Read the model definition and answer for the solid it produces. Units are mm, in the model's axes. A direction names the side the tool comes from. Give positions to 0.01 mm unless a question says otherwise; leave off trailing zeros. Order: outer loops, then holes, each group sorted by start corner. A loop starts at its lowest first (then second) coordinate and runs counter-clockwise, first axis right, second up. Notation, with made-up numbers: (35.25, 5.5) -> (89.25, 5.5) arc R25 cw to (89.25, 23.5) -> close; hole circle Ø10 at (5.5, 13). An arc over 180 degrees is marked (long way). Answer as CSV lines item,"result". Start each with the question number.
1) For faces 5 (the face through (-59.09, -59.46, 0.49)), 6 (the face through (-49, -57.4, 0.5)), determine the directions among +Z, -Z, +X, -X, +Y, -Y from which every point of the face is accessible in a straight line to the end or side of a thin tool.
2) Find section A-A (z = 0.15). State how many separate pieces and enclosed holes the cut face has, and give its area (3 significant figures).
3) The mould has two halves that part along Y. Classify faces 1 (the face through (59.328, -57.995, 0.493)), 2 (the face through (-49, -49.1, 0.5)), 3 (the face through (31, -48, 1)), 4 (the face through (-33, -49, 0.5)): +Y half, -Y half, draft (parallel to the pull), parting line (faces both ways), or undercut.
4) Find section C-C (y = -48). Determine the outline of the cut face in (x, z), and give its area (3 significant figures).
5) Find section D-D (x = 37). Determine the outline of the cut face in (y, z).
6) Flat-ended cylindrical pins translate along their axes: pin 1 Ø0.5 at (y, z) = (-46.5, 0.5) entering from +X; pin 2 Ø0.5 at (x, z) = (-15, 0.5) entering from -Y; pin 3 Ø0.5 at (y, z) = (-77.5, 0.5) entering from -X. Find the tip coordinate at first contact, or state that the pin passes through.
7) Find section B-B (y = -23). Determine the outline of the cut face in (x, z).
8) Straight lines are drawn through the part: L1, parallel to Y at x = -44, z = 0.25; L2, parallel to X at y = -48, z = 0.3; L3, parallel to X at y = -23.5, z = 0.9. For each, find the intervals that lie inside material, in ascending order. Write a range as from..to.
```python
from build123d import *

# Parameters (mm, degrees)
BOSS_EXTRUDE2_DEPTH = 1


with BuildPart() as part:
    # Sketch1 → Boss-Extrude2 (new body)
    with BuildSketch(Plane.XY):
        with BuildLine():
            Line((-30, -13.100406207), (-30, -101))
            ThreePointArc((-30, -101), (-59.212156956, -58.729733103), (-45, -9.352206107))
            Line((-45, -9.352206107), (45, -9.352206107))
            ThreePointArc((45, -9.352206107), (59.212156956, -58.729733103), (30, -101))
            Line((30, -101), (30, -13.100406207))
            Line((30, -13.100406207), (-30, -13.100406207))
        make_face()
        with BuildLine():
            Line((-35.65, -43.388475773), (-46.35, -43.388475773))
            ThreePointArc((-46.35, -43.388475773), (-49, -40.738475773), (-46.35, -38.088475773))
            Line((-46.35, -38.088475773), (-35.65, -38.088475773))
            ThreePointArc((-35.65, -38.088475773), (-33, -40.738475773), (-35.65, -43.388475773))
        make_face(mode=Mode.SUBTRACT)
        with BuildLine():
            Line((-35.65, -51.688475773), (-46.35, -51.688475773))
            ThreePointArc((-46.35, -51.688475773), (-49, -49.038475773), (-46.35, -46.388475773))
            Line((-46.35, -46.388475773), (-35.65, -46.388475773))
            ThreePointArc((-35.65, -46.388475773), (-33, -49.038475773), (-35.65, -51.688475773))
        make_face(mode=Mode.SUBTRACT)
        with BuildLine():
            Line((-35.65, -59.988475773), (-46.35, -59.988475773))
            ThreePointArc((-46.35, -59.988475773), (-49, -57.338475773), (-46.35, -54.688475773))
            Line((-46.35, -54.688475773), (-35.65, -54.688475773))
            ThreePointArc((-35.65, -54.688475773), (-33, -57.338475773), (-35.65, -59.988475773))
        make_face(mode=Mode.SUBTRACT)
        with BuildLine():
            Line((46.35, -43.388475773), (35.65, -43.388475773))
            ThreePointArc((35.65, -43.388475773), (33, -40.738475773), (35.65, -38.088475773))
            Line((35.65, -38.088475773), (46.35, -38.088475773))
            ThreePointArc((46.35, -38.088475773), (49, -40.738475773), (46.35, -43.388475773))
        make_face(mode=Mode.SUBTRACT)
        with BuildLine():
            Line((46.35, -51.688475773), (35.65, -51.688475773))
            ThreePointArc((35.65, -51.688475773), (33, -49.038475773), (35.65, -46.388475773))
            Line((35.65, -46.388475773), (46.35, -46.388475773))
            ThreePointArc((46.35, -46.388475773), (49, -49.038475773), (46.35, -51.688475773))
        make_face(mode=Mode.SUBTRACT)
        with BuildLine():
            Line((46.35, -59.988475773), (35.65, -59.988475773))
            ThreePointArc((35.65, -59.988475773), (33, -57.338475773), (35.65, -54.688475773))
            Line((35.65, -54.688475773), (46.35, -54.688475773))
            ThreePointArc((46.35, -54.688475773), (49, -57.338475773), (46.35, -59.988475773))
        make_face(mode=Mode.SUBTRACT)
    extrude(amount=BOSS_EXTRUDE2_DEPTH)


solid = part.part
```
Findings below:
1,face 5,"+Z, -Z, -X"
1,face 6,"+Z, -Z"
2,separate pieces,"1"
2,enclosed holes,"6"
2,area,"3,970 mm²"
3,face 1,"parting line"
3,face 2,"undercut"
3,face 3,"draft"
3,face 4,"undercut"
4,outline,"(-59.99, 0) -> (-48.79, 0) -> (-48.79, 1) -> (-59.99, 1) -> close; (-33.21, 0) -> (-30, 0) -> (-30, 1) -> (-33.21, 1) -> close; (30, 0) -> (33.21, 0) -> (33.21, 1) -> (30, 1) -> close; (48.79, 0) -> (59.99, 0) -> (59.99, 1) -> (48.79, 1) -> close"
4,area,"28.8 mm²"
5,outline,"(-96.27, 0) -> (-59.99, 0) -> (-59.99, 1) -> (-96.27, 1) -> close; (-54.69, 0) -> (-51.69, 0) -> (-51.69, 1) -> (-54.69, 1) -> close; (-46.39, 0) -> (-43.39, 0) -> (-43.39, 1) -> (-46.39, 1) -> close; (-38.09, 0) -> (-9.35, 0) -> (-9.35, 1) -> (-38.09, 1) -> close"
6,pin 1,"x = 59.96"
6,pin 2,"y = -13.1"
6,pin 3,"x = -52.95"
7,outline,"(-54.06, 0) -> (-30, 0) -> (-30, 1) -> (-54.06, 1) -> close; (30, 0) -> (54.06, 0) -> (54.06, 1) -> (30, 1) -> close"
8,L1,"-89.83..-59.99, -54.69..-51.69, -46.39..-43.39, -38.09..-9.35"
8,L2,"-59.99..-48.79, -33.21..-30, 30..33.21, 48.79..59.99"
8,L3,"-54.29..-30, 30..54.29"
